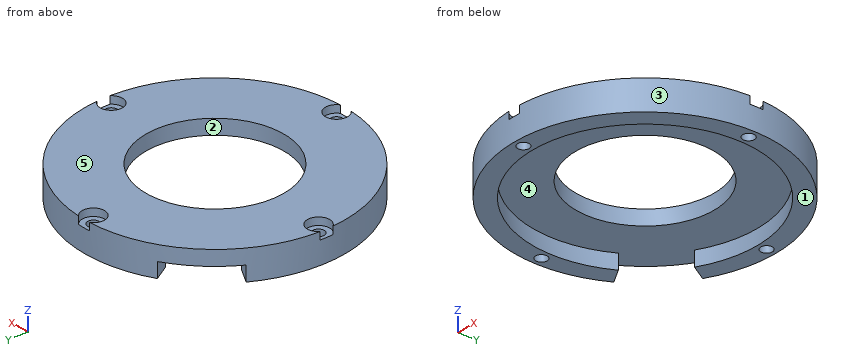
from build123d import *

# Parameters (mm, degrees)
EXTRUDE_1_OUTLINE_R   = 35
EXTRUDE_1_OUTLINE_R_2 = 1.55
EXTRUDE_1_OUTLINE_R_3 = 30.05
EXTRUDE_1_DEPTH       = 10
SKETCH_2_R            = 33.525
SKETCH_2_R_2          = 18.525
EXTRUDE_1_2_DEPTH     = 4
SKETCH_3_R            = 1.55
CUT_EXTRUDE_1_DEPTH   = 51.497524692
CUT_EXTRUDE_2_DEPTH   = 6
SKETCH_8_R            = 35
SKETCH_8_R_2          = 30.05
CUT_EXTRUDE_3_DEPTH   = 2
SKETCH_9_R            = 3
CUT_EXTRUDE_4_DEPTH   = 2


# Read off the part's stored shape, not the designer's step: 凸台-拉伸1
with BuildPart() as part:
    # Extrude 1 outline → Extrude 1 (new body)
    with BuildSketch(Plane.XY):
        Circle(EXTRUDE_1_OUTLINE_R)
        with Locations((0, -32.5)):
            Circle(EXTRUDE_1_OUTLINE_R_2, mode=Mode.SUBTRACT)
        with Locations((-32.5, 0)):
            Circle(EXTRUDE_1_OUTLINE_R_2, mode=Mode.SUBTRACT)
        Circle(EXTRUDE_1_OUTLINE_R_3, mode=Mode.SUBTRACT)
        with Locations((32.5, 0)):
            Circle(EXTRUDE_1_OUTLINE_R_2, mode=Mode.SUBTRACT)
        with Locations((0, 32.5)):
            Circle(EXTRUDE_1_OUTLINE_R_2, mode=Mode.SUBTRACT)
    extrude(amount=EXTRUDE_1_DEPTH)

    # 草图2 → Extrude 1 2 (add)
    with BuildSketch(Plane.XY.offset(10)):
        Circle(SKETCH_2_R)
        Circle(SKETCH_2_R_2, mode=Mode.SUBTRACT)
    extrude(amount=-EXTRUDE_1_2_DEPTH)

    # 草图3 → 切除-拉伸1 (cut, through all)
    with BuildSketch(Plane(origin=(0, 0, 0), x_dir=(-1, 0, 0), z_dir=(0, 0, -1))):
        with Locations(Location((32.5, 0, 0), (0, 0, 180))):
            Circle(SKETCH_3_R)
        with Locations(Location((0, -32.5, 0), (0, 0, 180))):
            Circle(SKETCH_3_R)
        with Locations(Location((-32.5, 0, 0), (0, 0, 180))):
            Circle(SKETCH_3_R)
        with Locations(Location((0, 32.5, 0), (0, 0, 180))):
            Circle(SKETCH_3_R)
    extrude(amount=-CUT_EXTRUDE_1_DEPTH, mode=Mode.SUBTRACT)

    # 草图7 → 切除-拉伸2 (cut)
    with BuildSketch(Plane(origin=(0, 0, 0), x_dir=(-1, 0, 0), z_dir=(0, 0, -1))):
        with BuildLine():
            Line((15.025, 26.024063384), (17.5, 30.310889132))
            ThreePointArc((17.5, 30.310889132), (24.748737342, 24.748737342), (30.310889132, 17.5))
            Line((30.310889132, 17.5), (26.024063384, 15.025))
            ThreePointArc((26.024063384, 15.025), (21.248558775, 21.248558775), (15.025, 26.024063384))
        make_face()
    extrude(amount=-CUT_EXTRUDE_2_DEPTH, mode=Mode.SUBTRACT)

    # 草图8 → 切除-拉伸3 (cut)
    with BuildSketch(Plane(origin=(0, 0, 0), x_dir=(-1, 0, 0), z_dir=(0, 0, -1))):
        with Locations(Location((0, 0, 0), (0, 0, 30))):
            Circle(SKETCH_8_R)
        Circle(SKETCH_8_R_2, mode=Mode.SUBTRACT)
    extrude(amount=-CUT_EXTRUDE_3_DEPTH, mode=Mode.SUBTRACT)

    # 草图9 → 切除-拉伸4 (cut)
    with BuildSketch(Plane.XY.offset(10)):
        with Locations((0, 32.5)):
            Circle(SKETCH_9_R)
        with Locations((32.5, 0)):
            Circle(SKETCH_9_R)
        with Locations((0, -32.5)):
            Circle(SKETCH_9_R)
        with Locations((-32.5, 0)):
            Circle(SKETCH_9_R)
    extrude(amount=-CUT_EXTRUDE_4_DEPTH, mode=Mode.SUBTRACT)


solid = part.part
Build history of the part. All positions in model axes, mm. Face numbers are marked on the shaded views. A direction names the side the tool comes from. Round coordinates to 2 decimals unless told otherwise and drop trailing zeros. Loops run counter-clockwise (first coordinate to the right, second up) from the corner with the lowest first, then second, coordinate; pieces in that order, holes last. Notation, with made-up numbers: (12, 0) -> (32, 0) arc R9 ccw to (32, 16) -> close; hole circle Ø9 at (-5, -0.5). An arc over 180 degrees is marked (long way). Answer in a Markdown table with one row per item.
Item 1: Mould opens along Y. For the marked faces 1, 2 and 3 say: +Y half, -Y half, draft (parallel to the pull), parting line (faces both ways), or undercut.
Answers below:
| item | result |
|---|---|
| face 1 | draft |
| face 2 | undercut |
| face 3 | parting line |
Item 2: Drill centre lines: L1, parallel to X at y = 0, z = 3.45; L2, parallel to Y at x = 0, z = 9.5 (3 decimals). Where is each one in solid material? Low to high. Write a range as [from, to].
Answers below:
| item | result |
|---|---|
| L1 | x = [-35, -34.05], [-30.95, -30.05], [30.05, 30.95], [34.05, 35] |
| L2 | y = [-29.5, -18.525], [18.525, 29.5] |
Item 3: Which spindle directions (+Z, -Z, +X, -X, +Y, -Y) get a long thin tool onto all of the face, cutting with end or side? Do the marked faces 4 and 5. Say none if no direction does.
Answers below:
| item | result |
|---|---|
| face 4 | -Z |
| face 5 | +Z, +X, -X, +Y, -Y |
Item 4: Saw through at A-A (y = 0). Write the cut outline in (x, z) (3 decimals), and give its area (3 significant figures).
Answers below:
| item | result |
|---|---|
| outline | (-35, 2) -> (-34.05, 2) -> (-34.05, 8) -> (-35, 8) -> close; (-30.95, 2) -> (-30.05, 2) -> (-30.05, 6) -> (-18.525, 6) -> (-18.525, 10) -> (-29.5, 10) -> (-29.5, 8) -> (-30.95, 8) -> close; (18.525, 6) -> (30.05, 6) -> (30.05, 2) -> (30.95, 2) -> (30.95, 8) -> (29.5, 8) -> (29.5, 10) -> (18.525, 10) -> close; (34.05, 2) -> (35, 2) -> (35, 8) -> (34.05, 8) -> close |
| area | 112 mm² |
Item 5: Pin check, flat tips, straight feed: pin 1 (2 mm diameter, centred on y = -3, z = 8, fed in from -X); pin 2 (4 mm diameter, centred on y = -7.5, z = 3, fed in from +X); pin 3 (4 mm diameter, centred on x = -32.5, y = 0, fed in from +Z); pin 4 (2.5 mm diameter, centred on x = 32.5, y = 0, fed in from +Z). Stop position of each tip, or through.
Answers below:
| item | result |
|---|---|
| pin 1 | stops at x = -34.94 |
| pin 2 | stops at x = 34.57 |
| pin 3 | stops at z = 8 |
| pin 4 | passes through |
Item 6: Saw through at C-C (z = 4.5). Write the cut outline in (x, y) (3 decimals).
Answers below:
| item | result |
|---|---|
| outline | (-30.311, 17.5) arc R35 ccw (long way) to (-17.5, 30.311) -> (-15.025, 26.024) arc R30.05 cw (long way) to (-26.024, 15.025) -> close; hole circle Ø3.1 at (-32.5, 0); hole circle Ø3.1 at (0, -32.5); hole circle Ø3.1 at (0, 32.5); hole circle Ø3.1 at (32.5, 0) |
Item 7: Saw through at D-D (x = 17.5). Write the cut outline in (y, z).
Answers below:
| item | result |
|---|---|
| outline | (-30.31, 2) -> (-24.43, 2) -> (-24.43, 6) -> (-6.08, 6) -> (-6.08, 10) -> (-30.31, 10) -> close; (6.08, 6) -> (24.43, 6) -> (24.43, 2) -> (30.31, 2) -> (30.31, 10) -> (6.08, 10) -> close |
